from build123d import *

# Parameters (mm, degrees)
F0_W     = 125.638232
F0_H     = 116.504982
F1_DEPTH = 50
F2_R     = 50.209764
F2_R_2   = 36.290229
F3_DEPTH = 25


with BuildPart() as f1:
    # F0 (on Front) → F1 (new body)
    with BuildSketch(Plane.XZ):
        Rectangle(F0_W, F0_H)
    extrude(amount=F1_DEPTH)

    # F2 (on face) → F3 (join)
    with BuildSketch(Plane.XZ.offset(50)):
        Circle(F2_R)
        Circle(F2_R_2, mode=Mode.SUBTRACT)
    extrude(amount=F3_DEPTH)


solid = f1.part
Input: part model. Units: mm. Frame: model coordinates. A direction names the side the tool comes from. Give positions to 0.01 mm unless a question says otherwise; leave off trailing zeros. Order: outer loops, then holes, each group sorted by start corner. A loop starts at its lowest first (then second) coordinate and runs counter-clockwise, first axis right, second up.
Q1. Section C-C on x = 0. Output: boundary loops of the cut face in (y, z).
Checked values:
outline: (-75, -50.21) - (-50, -50.21) - (-50, -58.25) - (0, -58.25) - (0, 58.25) - (-50, 58.25) - (-50, 50.21) - (-75, 50.21) - (-75, 36.29) - (-50, 36.29) - (-50, -36.29) - (-75, -36.29) - close
Q2. Section D-D on z = -39. Output: boundary loops of the cut face in (x, y), and give its area (3 significant figures).
Checked values:
outline: (-62.82, -50) - (-31.62, -50) - (-31.62, -75) - (31.62, -75) - (31.62, -50) - (62.82, -50) - (62.82, 0) - (-62.82, 0) - close
area: 7,860 mm2
Q3. Set-up query: faces 1 (the cylindrical face through (34.614, -62.325, 10.901)), 2 (the flat face through (33.2, -75, 15.1)). Return all of +Z, -Z, +X, -X, +Y, -Y with unobstructed straight access to the full face (end or side cutting, diameter ignored); none if empty.
Checked values:
face 1: -Y
face 2: +Z, -Z, +X, -X, -Y
Q4. Contact query for flat-ended pins moving along their axis: pin 1 Ø6 at (x, z) = (-30, -7.5) entering from +Y; pin 2 Ø3 at (y, z) = (-56.5, 46) entering from +X; pin 3 Ø3 at (x, y) = (-39, -59) entering from +Z; pin 4 Ø10 at (x, z) = (-7.5, 17.5) entering from -Y. Output: stop coordinate, or through.
Checked values:
pin 1: stops at y = 0
pin 2: stops at x = 23.25
pin 3: stops at z = 33.39
pin 4: stops at y = -50
Q5. Section A-A on z = 0. Output: boundary loops of the cut face in (x, y).
Checked values:
outline: (-62.82, -50) - (-50.21, -50) - (-50.21, -75) - (-36.29, -75) - (-36.29, -50) - (36.29, -50) - (36.29, -75) - (50.21, -75) - (50.21, -50) - (62.82, -50) - (62.82, 0) - (-62.82, 0) - close
Q6. Ray query, probe 1 along Z at (x, y) = (0, -64.25); probe 2 along Y at (x, z) = (24, 4); probe 3 along X at (y, z) = (-65, -1). Return the intervals inside material, ascending.
Checked values:
probe 1: z = -50.21 to -36.29, 36.29 to 50.21
probe 2: y = -50 to 0
probe 3: x = -50.2 to -36.28, 36.28 to 50.2
Q7. Draft query along X for faces 3 (the flat face through (-1, -50, 1)), 4 (the flat face through (-1, 0, 1)), 5 (the cylindrical face through (-39.845, -62.325, -30.552)). Return one class per face: +X half, -X half, draft (parallel to the pull), parting line (faces both ways), or undercut.
Checked values:
face 3: undercut
face 4: draft
face 5: parting line
Q8. Section B-B on y = -57. Output: boundary loops of the cut face in (x, z).
Checked values:
outline: circle Ø100.42 at (0, 0); hole circle Ø72.58 at (0, 0)
